Geometry: final body of the model. Coordinates: model frame, mm. A direction names the side the tool comes from. Coordinates: 2 decimals unless noted, no trailing zeros. Order: outer loops, then holes, each group sorted by start corner. A loop starts at its lowest first (then second) coordinate and runs counter-clockwise, first axis right, second up. Notation, with made-up numbers: (13, 74) - (24, 74) arc R37 cw to (24, 113) - close; hole circle Ø6 at (32.5, -2). An arc over 180 degrees is marked (long way). Use one line per item in the form item = value. Start each with the question number.
```python
from build123d import *

# Parameters (mm, degrees)
SKETCH1_W                   = 20
SKETCH1_H                   = 17
BOSS_EXTRUDE1_DEPTH         = 4
SKETCH2_W                   = 20
SKETCH2_H                   = 37
BOSS_EXTRUDE2_DEPTH         = 15
M5_TAPPED_HOLE1_D           = 4.2
M5_TAPPED_HOLE1_DEPTH       = 9.8
M5_TAPPED_HOLE1_CSINK_D     = 5.05
M5_TAPPED_HOLE1_CSINK_ANGLE = 90
M5_TAPPED_HOLE1_TIP         = 1.2618073
SKETCH5_R                   = 3.05
CUT_EXTRUDE1_DEPTH          = 25
CHAMFER1_SIZE               = 6


with BuildPart() as part:
    # Sketch1 → Boss-Extrude1 (new body)
    with BuildSketch(Plane.XY):
        Rectangle(SKETCH1_W, SKETCH1_H)
    extrude(amount=BOSS_EXTRUDE1_DEPTH)

    # Sketch2 → Boss-Extrude2 (add)
    with BuildSketch(Plane(origin=(0, 0, 0), x_dir=(-1, 0, 0), z_dir=(0, 0, -1))):
        with Locations((0, 10)):
            Rectangle(SKETCH2_W, SKETCH2_H)
    extrude(amount=BOSS_EXTRUDE2_DEPTH)

    # M5 Tapped Hole1
    with Locations(Plane(origin=(0, 16.5, 0), x_dir=(1, 0, 0), z_dir=(0, 0, 1))):
        with Locations((0, 0)):
            CounterSinkHole(M5_TAPPED_HOLE1_D / 2, M5_TAPPED_HOLE1_CSINK_D / 2, depth=M5_TAPPED_HOLE1_DEPTH, counter_sink_angle=M5_TAPPED_HOLE1_CSINK_ANGLE)
            with Locations((0, 0, -(M5_TAPPED_HOLE1_DEPTH + M5_TAPPED_HOLE1_TIP / 2))):  # 118° drill point
                Cone(0, M5_TAPPED_HOLE1_D / 2, M5_TAPPED_HOLE1_TIP, mode=Mode.SUBTRACT)

    # Sketch5 → Cut-Extrude1 (cut)
    with BuildSketch(Plane.XZ.offset(8.5)):
        with Locations(Location((0, -5, 0), (0, 0, 270))):
            Circle(SKETCH5_R)
    extrude(amount=-CUT_EXTRUDE1_DEPTH, mode=Mode.SUBTRACT)

    # Chamfer1
    chamfer1_edges = [part.edges().sort_by_distance(p)[0] for p in [
        (10, 10, -15),
        (-10, 10, -15),
    ]]
    chamfer(chamfer1_edges, length=CHAMFER1_SIZE)


solid = part.part
```
(1) Cut plane B-B on x = -5.5. Return the cut outline in (y, z), plus the area to 4 significant figures.
(2) Contact query for flat-ended pins moving along their axis: pin 1 Ø4.5 at (x, z) = (-1, 1.5) entering from +Y; pin 2 Ø2 at (x, y) = (-6, 10.5) entering from +Z. Output: stop coordinate, or through.
(3) Draft query along Y for faces 1 (the flat face through (0, 28.5, -7)), 2 (the flat face through (-7, 10, -12)), 3 (the conical face through (-0.047, 16.862, -10.843)). Return one class per face: released by +Y, released by -Y, zero draft, split by the parting line, or undercut.
(4) Cut plane C-C on z = -4.75. Return the cut outline in (x, y).
(5) Set-up query: faces 4 (the flat face through (0, 21, 0)), 5 (the flat face through (0, 0, 4)), 6 (the cylindrical face through (0.134, 3.825, -1.953)), 7 (the cylindrical face through (0.273, 18.582, -5.178)). Return all of +Z, -Z, +X, -X, +Y, -Y with unobstructed straight access to the full face (end or side cutting, diameter ignored); none if empty.
(6) Cut plane D-D on y = 24.5. Return the cut outline in (x, z), plus the area to 3 significant figures.
(7) Cut plane A-A on z = -1. Return the cut outline in (x, y).
(8) Material intervals for L1, parallel to X at y = 5, z = -5; L2, parallel to Z at x = 0, y = 10.5; L3, parallel to Z at x = 0, y = 5, sorted ascending. Write a range as from..to.
Check sheet entries:
q1.outline = (-8.5, -13.5) - (28.5, -13.5) - (28.5, 0) - (8.5, 0) - (8.5, 4) - (-8.5, 4) - close
q1.area = 567.5 mm^2
q2.pin_1 = 28.5
q2.pin_2 = 0
q3.face_1 = released by +Y
q3.face_2 = zero draft
q3.face_3 = undercut
q4.outline = (-10, -8.5) - (-3.04, -8.5) - (-3.04, 16.5) - (-2.1, 16.5) arc R2.1 cw to (2.1, 16.5) - (3.04, 16.5) - (3.04, -8.5) - (10, -8.5) - (10, 28.5) - (-10, 28.5) - close
q5.face_4 = +Z, +X, -X, +Y
q5.face_5 = +Z, +X, -X, +Y, -Y
q5.face_6 = -Y
q5.face_7 = +Z
q6.outline = (-10, -9) - (-4, -15) - (4, -15) - (10, -9) - (10, 0) - (-10, 0) - close
q6.area = 264 mm^2
q7.outline = (-10, -8.5) - (10, -8.5) - (10, 28.5) - (-10, 28.5) - close; hole circle Ø4.2 at (0, 16.5)
q8.L1 = -10..-3.05, 3.05..10
q8.L2 = -15..-8.05, -1.95..0
q8.L3 = -15..-8.05, -1.95..4
